Geometry: final body of the model. Coordinates: model frame, mm. A direction names the side the tool comes from. Give positions to 0.01 mm unless a question says otherwise; leave off trailing zeros. Order: outer loops, then holes, each group sorted by start corner. A loop starts at its lowest first (then second) coordinate and runs counter-clockwise, first axis right, second up. Notation, with made-up numbers: (12, 60.25) -> (24, 60.25) arc R23 ccw to (24, 68.25) -> close; hole circle Ø9 at (0, 5.5). An arc over 180 degrees is marked (long way). Write item = value, one per line.
```python
from build123d import *

# Parameters (mm, degrees)
F1_DEPTH = 31.75
F2_W     = 76.2
F2_H     = 63.5
F3_DEPTH = 6.35
F4_W     = 76.2
F4_H     = 63.5
F5_DEPTH = 6.35


with BuildPart() as f1:
    # F0 (on Top) → F1 (new body, symmetric)
    with BuildSketch(Plane.XY):
        Polygon((1828.8, 31.75), (0, 31.75), (0, 28.575), (1825.625, 28.575), (1825.625, -28.575), (0, -28.575), (0, -31.75), (1828.8, -31.75), align=None)
    extrude(amount=F1_DEPTH, both=True)

    # F2 (on face) → F3 (join)
    with BuildSketch(Plane(origin=(0, 0, -31.75), x_dir=(1, 0, 0), z_dir=(0, 0, -1))):
        with Locations((1790.7, 0)):
            Rectangle(F2_W, F2_H)
    extrude(amount=F3_DEPTH)

    # F4 (on face) → F5 (join)
    with BuildSketch(Plane.XY.offset(31.75)):
        with Locations((1790.7, 0)):
            Rectangle(F4_W, F4_H)
    extrude(amount=F5_DEPTH)


solid = f1.part
```
1) Mould query, pull axis Z, two halves, no side actions, for faces 3 (the face through (1789, 0, 31.75)), 4 (the face through (902, -31.75, -1)), 5 (the face through (1790, 0, 38.1)), 6 (the face through (1789, 0, -31.75)). Classes: +Z half, -Z half, draft (parallel to the pull), parting line (faces both ways), or undercut.
Check sheet entries:
face_3 = undercut
face_4 = draft
face_5 = +Z half
face_6 = undercut
2) Section query A-A (x = 818). Output: boundary loops of the cut face in (y, z) (3 decimals).
Check sheet entries:
outline = (-31.75, -31.75) -> (-28.575, -31.75) -> (-28.575, 31.75) -> (-31.75, 31.75) -> close; (28.575, -31.75) -> (31.75, -31.75) -> (31.75, 31.75) -> (28.575, 31.75) -> close
3) Line query: line 1 (Y direction, x = 1189.5, z = 4.5) (3 decimals); line 2 (Z direction, x = 1509, y = 29); line 3 (X direction, y = -7.5, z = 17.5) (3 decimals). Output: solid intervals per line, ascending. Write a range as from..to.
Check sheet entries:
line_1 = -31.75..-28.575, 28.575..31.75
line_2 = -31.75..31.75
line_3 = 1825.625..1828.8
4) Section query C-C (z = -15). Output: boundary loops of the cut face in (x, y) (3 decimals).
Check sheet entries:
outline = (0, -31.75) -> (1828.8, -31.75) -> (1828.8, 31.75) -> (0, 31.75) -> (0, 28.575) -> (1825.625, 28.575) -> (1825.625, -28.575) -> (0, -28.575) -> close
5) First-contact query: P1, Ø3, axis at y = -14.5, z = 36.5, coming from the -X side; P2, Ø1, axis at x = 972, y = -31, coming from the +Z side; P3, Ø12, axis at y = 2, z = 4, coming from the -X side (3 decimals). Flat tips, straight axial feed; report the tip coordinate or a pass-through.
Check sheet entries:
P1 = 1752.6
P2 = 31.75
P3 = 1825.625
6) Reachability of faces 1 (the face through (1828.8, 0, -1)), 2 (the face through (1825.625, 0, 0)) from +Z, -Z, +X, -X, +Y, -Y: full face, straight path, thin tool, end or side. Return the list, or none.
Check sheet entries:
face_1 = +Z, -Z, +X, +Y, -Y
face_2 = -X
7) Section query B-B (y = 16). Output: boundary loops of the cut face in (x, z) (3 decimals), plus the area to 3 significant figures.
Check sheet entries:
outline = (1752.6, -38.1) -> (1828.8, -38.1) -> (1828.8, 38.1) -> (1752.6, 38.1) -> (1752.6, 31.75) -> (1825.625, 31.75) -> (1825.625, -31.75) -> (1752.6, -31.75) -> close
area = 1,170 mm²
